Can you work these out from the model? Positions are in its coordinate system, mm. Give positions to 0.01 mm unless a question says otherwise; leave off trailing zeros. Loops run counter-clockwise (first coordinate to the right, second up) from the corner with the lowest first, then second, coordinate; pieces in that order, holes last. Notation, with made-up numbers: M 66,2 L 71,2 A30 cw 71,40 Z; hole C 7.5,31 d11. An arc over 180 degrees is marked long. Answer as a JSON object with one key per item and string values.
```python
from build123d import *

# Parameters (mm, degrees)
SKETCH1_W                    = 184
SKETCH1_H                    = 18
BOSS_EXTRUDE1_DEPTH          = 658
F_3_0_3_DIAMETER_HOLE2_D     = 3
F_3_0_3_DIAMETER_HOLE2_DEPTH = 5
F_3_0_3_DIAMETER_HOLE2_TIP   = 0.901290929
CUT_EXTRUDE3_DEPTH           = 16
CAVITY1_START                = -640
CAVITY1_DEPTH                = 10
CAVITY1_START_2              = -10
CAVITY1_2_DEPTH              = 10


# Read off the part's stored shape, not the designer's step: Cavity1
with BuildPart() as part:
    # Sketch1 → Boss-Extrude1 (new body)
    with BuildSketch(Plane.XY):
        with Locations((-97.838367622, -1030.94)):
            Rectangle(SKETCH1_W, SKETCH1_H)
    extrude(amount=-BOSS_EXTRUDE1_DEPTH)

    # Ø3.0 (3) Diameter Hole2
    with Locations(Plane(origin=(0, -1039.94, 0), x_dir=(-1, 0, 0), z_dir=(0, -1, 0))):
        with Locations((97.838367622, 64), (97.838367622, 384), (97.838367622, 576), (97.838367622, 192), (97.838367622, 15.63)):
            Hole(F_3_0_3_DIAMETER_HOLE2_D / 2, depth=F_3_0_3_DIAMETER_HOLE2_DEPTH)
            with Locations((0, 0, -(F_3_0_3_DIAMETER_HOLE2_DEPTH + F_3_0_3_DIAMETER_HOLE2_TIP / 2))):  # 118° drill point
                Cone(0, F_3_0_3_DIAMETER_HOLE2_D / 2, F_3_0_3_DIAMETER_HOLE2_TIP, mode=Mode.SUBTRACT)

    # Sketch8 → Cut-Extrude3 (cut)
    with BuildSketch(Plane.XZ.offset(1039.94)):
        with BuildLine():
            Line((-108.088367622, -85.802173793), (-108.088367622, -74.197826207))
            ThreePointArc((-108.088367622, -74.197826207), (-106.088367622, -72.197826207), (-104.088367622, -74.197826207))
            Line((-104.088367622, -74.197826207), (-104.088367622, -85.802173793))
            ThreePointArc((-104.088367622, -85.802173793), (-106.088367622, -87.802173793), (-108.088367622, -85.802173793))
        make_face()
        with BuildLine():
            Line((-108.088367622, -373.121722836), (-108.088367622, -362.878277164))
            ThreePointArc((-108.088367622, -362.878277164), (-106.088367622, -360.878277164), (-104.088367622, -362.878277164))
            Line((-104.088367622, -362.878277164), (-104.088367622, -373.121722836))
            ThreePointArc((-104.088367622, -373.121722836), (-106.088367622, -375.121722836), (-108.088367622, -373.121722836))
        make_face()
        with BuildLine():
            Line((-108.088367622, -565.121722836), (-108.088367622, -554.878277164))
            ThreePointArc((-108.088367622, -554.878277164), (-106.088367622, -552.878277164), (-104.088367622, -554.878277164))
            Line((-104.088367622, -554.878277164), (-104.088367622, -565.121722836))
            ThreePointArc((-104.088367622, -565.121722836), (-106.088367622, -567.121722836), (-108.088367622, -565.121722836))
        make_face()
    extrude(amount=-CUT_EXTRUDE3_DEPTH, mode=Mode.SUBTRACT)

    # Cavity1 outline → Cavity1 (cut)
    with BuildSketch(Plane.XY.offset(CAVITY1_START)):
        with BuildLine():
            Line((-150.838367622, -1039.94), (-150.838367622, -1027.182640687))
            ThreePointArc((-150.838367622, -1027.182640687), (-150.838367621, -1022.94), (-146.595726934, -1022.94))
            Line((-146.595726934, -1022.94), (-120.081008309, -1022.94))
            ThreePointArc((-120.081008309, -1022.94), (-115.838367622, -1022.94), (-115.838367622, -1027.182640687))
            Line((-115.838367622, -1027.182640687), (-115.838367622, -1039.94))
            Line((-115.838367622, -1039.94), (-79.838367622, -1039.94))
            Line((-79.838367622, -1039.94), (-79.838367622, -1027.182640687))
            ThreePointArc((-79.838367622, -1027.182640687), (-79.838367621, -1022.94), (-75.595726934, -1022.94))
            Line((-75.595726934, -1022.94), (-49.081008309, -1022.94))
            ThreePointArc((-49.081008309, -1022.94), (-44.838367622, -1022.94), (-44.838367622, -1027.182640687))
            Line((-44.838367622, -1027.182640687), (-44.838367622, -1039.94))
            Line((-44.838367622, -1039.94), (-5.838367622, -1039.94))
            Line((-5.838367622, -1039.94), (-5.838367622, -1021.94))
            Line((-5.838367622, -1021.94), (-189.838367622, -1021.94))
            Line((-189.838367622, -1021.94), (-189.838367622, -1039.94))
            Line((-189.838367622, -1039.94), (-150.838367622, -1039.94))
        make_face()
    extrude(amount=CAVITY1_DEPTH, mode=Mode.SUBTRACT)

    # Cavity1 2 outline → Cavity1 2 (cut)
    with BuildSketch(Plane.XY.offset(CAVITY1_START_2)):
        with BuildLine():
            Line((-150.838367622, -1039.94), (-150.838367622, -1027.182640687))
            ThreePointArc((-150.838367622, -1027.182640687), (-150.838367621, -1022.94), (-146.595726934, -1022.94))
            Line((-146.595726934, -1022.94), (-120.081008309, -1022.94))
            ThreePointArc((-120.081008309, -1022.94), (-115.838367622, -1022.94), (-115.838367622, -1027.182640687))
            Line((-115.838367622, -1027.182640687), (-115.838367622, -1039.94))
            Line((-115.838367622, -1039.94), (-79.838367622, -1039.94))
            Line((-79.838367622, -1039.94), (-79.838367622, -1027.182640687))
            ThreePointArc((-79.838367622, -1027.182640687), (-79.838367621, -1022.94), (-75.595726934, -1022.94))
            Line((-75.595726934, -1022.94), (-49.081008309, -1022.94))
            ThreePointArc((-49.081008309, -1022.94), (-44.838367622, -1022.94), (-44.838367622, -1027.182640687))
            Line((-44.838367622, -1027.182640687), (-44.838367622, -1039.94))
            Line((-44.838367622, -1039.94), (-5.838367622, -1039.94))
            Line((-5.838367622, -1039.94), (-5.838367622, -1021.94))
            Line((-5.838367622, -1021.94), (-189.838367622, -1021.94))
            Line((-189.838367622, -1021.94), (-189.838367622, -1039.94))
            Line((-189.838367622, -1039.94), (-150.838367622, -1039.94))
        make_face()
    extrude(amount=CAVITY1_2_DEPTH, mode=Mode.SUBTRACT)


solid = part.part
```
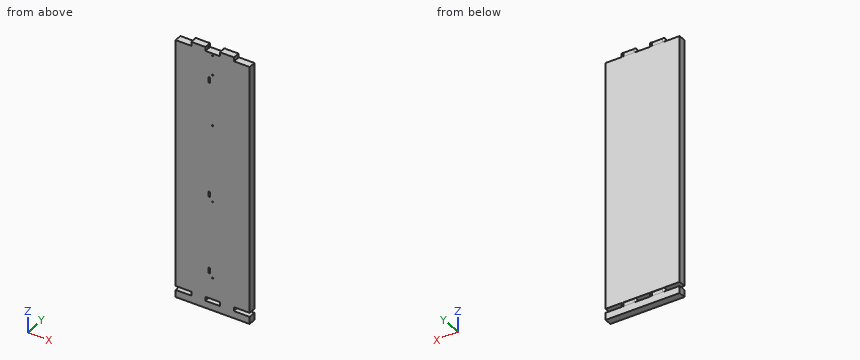
1) Will these pins go through, and if not, where does the flat tip stop? pin 1 Ø5 at (y, z) = (-1036, -3) entering from -X; pin 2 Ø3 at (x, z) = (-137, -635.5) entering from +Y; pin 3 Ø2.5 at (x, z) = (-97.84, -15.63) entering from -Y.
Answer list:
{"pin 1": "x = -150.84", "pin 2": "y = -1022.94", "pin 3": "y = -1034.79"}
2) Please list where these lines run through material, in increasing order: line 1 along Z through (x, y) = (-170.5, -1023.5); line 2 along X through (y, z) = (-1036, -192). Write a range as from..to.
Answer list:
{"line 1": "-658..-640, -630..-10", "line 2": "-189.84..-99.34, -96.34..-5.84"}
3) Suppose I cut it at A-A, the plane x = -21. Write out the boundary of the cut face in (y, z).
Answer list:
{"outline": "M -1039.94,-658 L -1021.94,-658 L -1021.94,-640 L -1039.94,-640 Z; M -1039.94,-630 L -1021.94,-630 L -1021.94,-10 L -1039.94,-10 Z"}
4) Suppose I cut it at B-B, the plane y = -1031. Give the number of separate pieces and of enclosed holes in the cut face, and give its area (3 significant figures).
Answer list:
{"separate pieces": "1", "enclosed holes": "4", "area": "119,000 mm^2"}
